Drawing for the job (mm, zero at the part's lowest x, y, z). A direction names the side the tool comes from. Give positions to 0.01 mm unless a question says otherwise; leave off trailing zeros. Write each loop counter-clockwise with the first axis right and the second up, starting at its lowest first coordinate (ties: lowest second). Pieces come first, ordered by that corner, then holes.
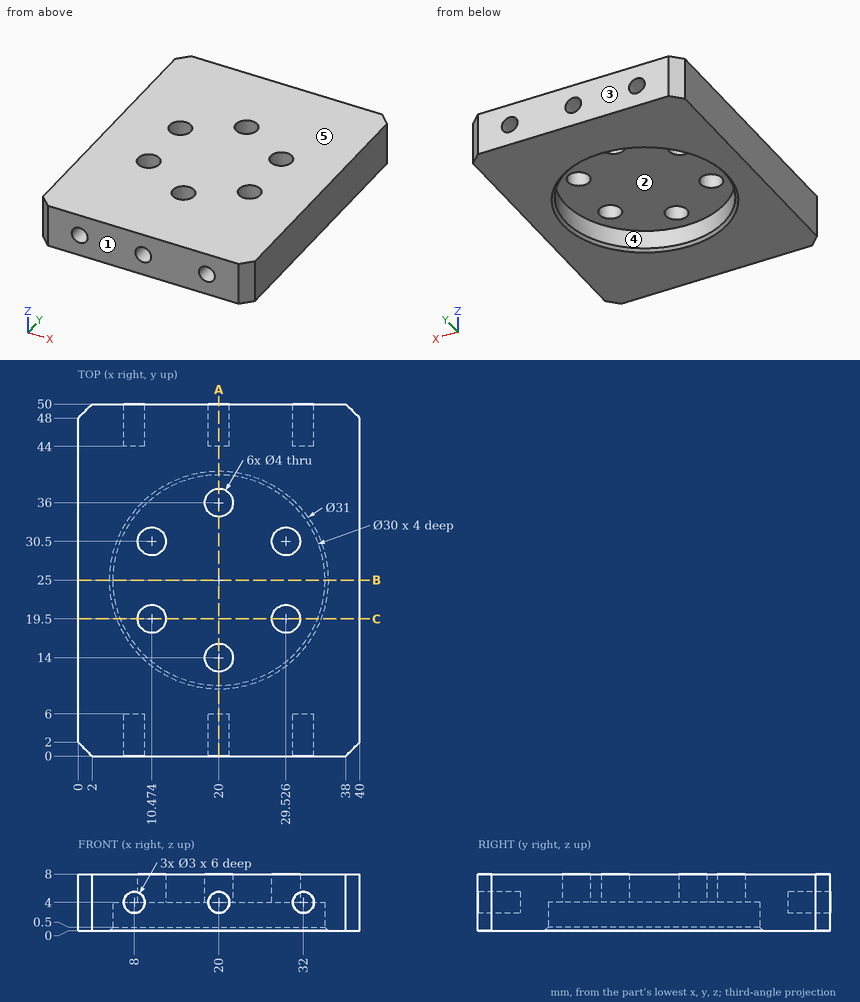
1. Slice it at C-C, the plane y = 19.5. State how many separate pieces and enclosed holes the cut face has, and give its area (3 significant figures).
Calculated:
separate pieces: 3
enclosed holes: 0
area: 176 mm2
2. Probe probe 1 along Y at (x, z) = (10, 6); probe 2 along X at (y, z) = (2, 4); probe 3 along Z at (x, y) = (32, 1.65). List the from-to ranges inside material, lowest first.
Calculated:
probe 1: y = 0 to 17.56, 21.44 to 28.56, 32.44 to 50
probe 2: x = 0 to 6.5, 9.5 to 18.5, 21.5 to 30.5, 33.5 to 40
probe 3: z = 0 to 2.5, 5.5 to 8
3. Slice it at B-B, the plane y = 25. Write the cut outline in (x, z), and give its area (3 significant figures).
Calculated:
outline: (0, 0) - (4.5, 0) - (5, 0.5) - (5, 4) - (35, 4) - (35, 0.5) - (35.5, 0) - (40, 0) - (40, 8) - (0, 8) - close
area: 200 mm2
4. Slice it at A-A, the plane x = 20. Write the cut outline in (y, z), and give its area (3 significant figures).
Calculated:
outline: (0, 0) - (9.5, 0) - (10, 0.5) - (10, 4) - (12, 4) - (12, 8) - (0, 8) - (0, 5.5) - (6, 5.5) - (6, 2.5) - (0, 2.5) - close; (16, 4) - (34, 4) - (34, 8) - (16, 8) - close; (38, 4) - (40, 4) - (40, 0.5) - (40.5, 0) - (50, 0) - (50, 2.5) - (44, 2.5) - (44, 5.5) - (50, 5.5) - (50, 8) - (38, 8) - close
area: 212 mm2
5. Pull direction Y, two halves, no side cores. Call the marked faces 3, 4 and 5: +Y half, -Y half, draft (parallel to the pull), parting line (faces both ways), or undercut.
Calculated:
face 3: +Y half
face 4: undercut
face 5: draft
6. Pin check, flat tips, straight feed: P1, Ø3.5, axis at x = 19.5, z = 4, coming from the +Y side; P2, Ø3, axis at x = 23, y = 30.5, coming from the -Z side; P3, Ø0.9, axis at x = 20, z = 4, coming from the -Y side; P4, Ø0.9, axis at x = 7.5, z = 4, coming from the +Y side. Stop position of each tip, or through.
Calculated:
P1: stops at y = 50
P2: stops at z = 4
P3: stops at y = 6
P4: stops at y = 44
7. Which spindle directions (+Z, -Z, +X, -X, +Y, -Y) get a long thin tool onto all of the face, cutting with end or side? Do the marked faces 1 and 2. Say none if no direction does.
Calculated:
face 1: +Z, -Z, +X, -X, -Y
face 2: -Z
